Work out the finished part from the listing and answer in its coordinate system (mm). Face numbers are marked on the shaded views. A direction names the side the tool comes from. Give positions to 0.01 mm unless a question says otherwise; leave off trailing zeros. Loops run counter-clockwise (first coordinate to the right, second up) from the corner with the lowest first, then second, coordinate; pieces in that order, holes last. Notation, with made-up numbers: (-9.75, 51.5) -> (8.25, 51.5) arc R20 cw to (8.25, 70.5) -> close; hole circle Ø10 at (-30.5, 30). An arc over 180 degrees is marked (long way). Answer as CSV lines item,"result". Start each with the question number.
1. Flat-ended cylindrical pins translate along their axes: pin 1 Ø1.5 at (x, z) = (-14, -12) entering from -Y; pin 2 Ø4 at (y, z) = (3, 3.5) entering from -X; pin 3 Ø2 at (y, z) = (4.5, 10.5) entering from -X; pin 4 Ø10 at (y, z) = (22, 3) entering from -X. Find the tip coordinate at first contact, or state that the pin passes through.
2. Determine the mould class of the marked faces 3, 4 and 5 for opening direction X: +X half, -X half, draft (parallel to the pull), parting line (faces both ways), or undercut.
3. Find section A-A, the plane y = 21.5. Give the vertices of the cut face in (x, z).
4. A tool of negligible diameter and unlimited length cuts with its end or side. For the marked faces 1 and 2, from which of +Z, -Z, +X, -X, +Y, -Y can it reach the whole face along a straight path? Write none if from no direction.
5. Find the intervals of material crossed by line 1 along Z through (x, y) = (0, 20); line 2 along Z through (x, y) = (0, 16.75); line 3 along Y through (x, z) = (-12, -2.5), in increasing order.
6. Find section B-B, the plane y = 11. Give the vertices of the cut face in (x, z), and give its area (3 significant figures).
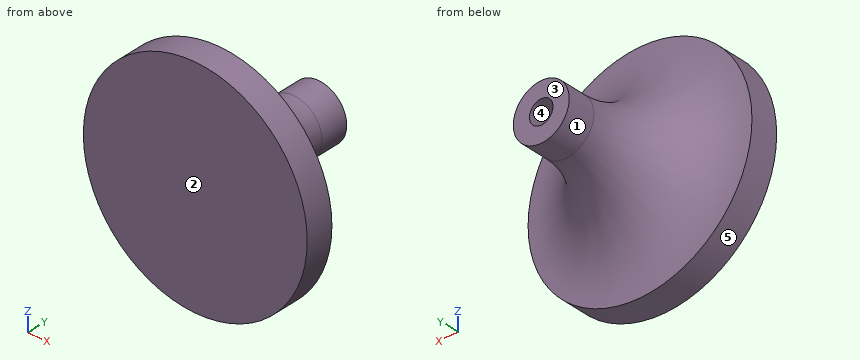
from build123d import *

# Parameters (mm, degrees)
M5X0_8_TAPPED_HOLE1_D     = 4.2
M5X0_8_TAPPED_HOLE1_DEPTH = 19
M5X0_8_TAPPED_HOLE1_TIP   = 1.2618073


with BuildPart() as part:
    # Sketch2 → Revolve1 (revolve)
    with BuildSketch(Plane.XY):
        with BuildLine():
            Line((0, 0), (-20, 0))
            Line((-20, 0), (-20, 5))
            ThreePointArc((-20, 5), (-9.393398282, 9.393398282), (-5, 20))
            Line((-5, 20), (-5, 25))
            Line((-5, 25), (0, 25))
            Line((0, 25), (0, 0))
        make_face()
    revolve(axis=Axis((0, 25, 0), (0, -1, 0)))

    # M5x0.8 Tapped Hole1
    with Locations(Plane(origin=(0, 25, 0), x_dir=(1, 0, 0), z_dir=(0, 1, 0))):
        with Locations((0, 0)):
            Hole(M5X0_8_TAPPED_HOLE1_D / 2, depth=M5X0_8_TAPPED_HOLE1_DEPTH)
            with Locations((0, 0, -(M5X0_8_TAPPED_HOLE1_DEPTH + M5X0_8_TAPPED_HOLE1_TIP / 2))):  # 118° drill point
                Cone(0, M5X0_8_TAPPED_HOLE1_D / 2, M5X0_8_TAPPED_HOLE1_TIP, mode=Mode.SUBTRACT)


solid = part.part
Resolved:
1,pin 1,"stops at y = 0"
1,pin 2,"stops at x = -19.94"
1,pin 3,"stops at x = -17.6"
1,pin 4,"stops at x = -5.16"
2,face 3,"draft"
2,face 4,"undercut"
2,face 5,"parting line"
3,outline,"circle Ø10 at (0, 0); hole circle Ø4.2 at (0, 0)"
4,face 1,"+Y"
4,face 2,"+Z, -Z, +X, -X, -Y"
5,line 1,"z = -5 to -2.1, 2.1 to 5"
5,line 2,"z = -5.36 to -2.1, 2.1 to 5.36"
5,line 3,"y = 0 to 7.15"
6,outline,"circle Ø16 at (0, 0); hole circle Ø4.2 at (0, 0)"
6,area,"187 mm^2"
